from build123d import *

# Parameters (mm, degrees)
SKETCH1_R            = 10
BOSS_EXTRUDE1_DEPTH  = 340
SKETCH2_R            = 5
CUT_EXTRUDE1_DEPTH   = 330
BOSS_EXTRUDE2_START  = -10
SKETCH3_R            = 10
BOSS_EXTRUDE2_DEPTH  = 50
BOSS_EXTRUDE3_DEPTH  = 10
BOSS_EXTRUDE4_START  = -40
BOSS_EXTRUDE4_DEPTH  = 10
BOSS_EXTRUDE6_START  = 10
SKETCH5_W            = 35
SKETCH5_H            = 30
BOSS_EXTRUDE6_DEPTH  = 10
SKETCH6_W            = 35
SKETCH6_H            = 30
BOSS_EXTRUDE8_DEPTH  = 11
SKETCH7_R            = 6
CUT_EXTRUDE2_DEPTH   = 21
SKETCH8_R            = 2.5
BOSS_EXTRUDE9_DEPTH  = 4
SKETCH9_R            = 10
SKETCH9_R_2          = 7.5
SKETCH9_R_3          = 2.5
CUT_EXTRUDE3_DEPTH   = 3
SKETCH10_R           = 2
BOSS_EXTRUDE10_DEPTH = 5


with BuildPart() as part:
    # Sketch1 → Boss-Extrude1 (new body)
    with BuildSketch(Plane.XY):
        Circle(SKETCH1_R)
    extrude(amount=BOSS_EXTRUDE1_DEPTH)

    # Sketch2 → Cut-Extrude1 (cut)
    with BuildSketch(Plane.XY.offset(340)):
        Circle(SKETCH2_R)
    extrude(amount=-CUT_EXTRUDE1_DEPTH, mode=Mode.SUBTRACT)

    # Sketch3 → Boss-Extrude2 (add)
    with BuildSketch(Plane(origin=(0, 0, 0), x_dir=(-1, 0, 0), z_dir=(0, 0, -1)).offset(BOSS_EXTRUDE2_START)):
        Polygon((17.320508076, 0), (8.660254038, 15), (-8.660254038, 15), (-17.320508076, 0), (-8.660254038, -15), (8.660254038, -15), align=None)
        Circle(SKETCH3_R, mode=Mode.SUBTRACT)
    extrude(amount=-BOSS_EXTRUDE2_DEPTH)

    # Sketch4 → Boss-Extrude3 (add)
    with BuildSketch(Plane(origin=(0, 0, 10), x_dir=(-1, 0, 0), z_dir=(0, 0, -1))):
        Polygon((-9.526279442, -16.5), (9.526279442, -16.5), (19.052558883, 0), (9.526279442, 16.5), (-9.526279442, 16.5), (-19.052558883, 0), align=None)
        Polygon((8.660254038, 15), (-8.660254038, 15), (-17.320508076, 0), (-8.660254038, -15), (8.660254038, -15), (17.320508076, 0), align=None, mode=Mode.SUBTRACT)
    extrude(amount=-BOSS_EXTRUDE3_DEPTH)

    # Sketch4_2 → Boss-Extrude4 (add)
    with BuildSketch(Plane(origin=(0, 0, 10), x_dir=(-1, 0, 0), z_dir=(0, 0, -1)).offset(BOSS_EXTRUDE4_START)):
        Polygon((-9.526279442, -16.5), (9.526279442, -16.5), (19.052558883, 0), (9.526279442, 16.5), (-9.526279442, 16.5), (-19.052558883, 0), align=None)
        Polygon((8.660254038, 15), (-8.660254038, 15), (-17.320508076, 0), (-8.660254038, -15), (8.660254038, -15), (17.320508076, 0), align=None, mode=Mode.SUBTRACT)
    extrude(amount=-BOSS_EXTRUDE4_DEPTH)



with BuildPart() as body_2:
    # Sketch5 → Boss-Extrude6 (new body)
    with BuildSketch(Plane(origin=(10, 0, 0), x_dir=(0, 0, -1), z_dir=(1, 0, 0)).offset(BOSS_EXTRUDE6_START)):
        with Locations((-77.5, 1.5)):
            Rectangle(SKETCH5_W, SKETCH5_H)
    extrude(amount=BOSS_EXTRUDE6_DEPTH)


with BuildPart() as part_1:
    add(part.part)

    add(body_2.part)  # Boss-Extrude8 merges body 2
    # Sketch6 → Boss-Extrude8 (add)
    with BuildSketch(Plane.ZY.offset(-20)):
        with Locations((77.5, 1.5)):
            Rectangle(SKETCH6_W, SKETCH6_H)
    extrude(amount=BOSS_EXTRUDE8_DEPTH)

    # Sketch7 → Cut-Extrude2 (cut)
    with BuildSketch(Plane(origin=(0, 16.5, 0), x_dir=(1, 0, 0), z_dir=(0, 1, 0))):
        with Locations((19.5, -85)):
            Circle(SKETCH7_R)
    extrude(amount=-CUT_EXTRUDE2_DEPTH, mode=Mode.SUBTRACT)

    # Sketch8 → Boss-Extrude9 (add)
    with BuildSketch(Plane.ZY.offset(-9)):
        with Locations((90, 11.5)):
            Circle(SKETCH8_R)
    extrude(amount=BOSS_EXTRUDE9_DEPTH)

    # Sketch9 → Cut-Extrude3 (cut)
    with BuildSketch(Plane(origin=(30, 0, 0), x_dir=(0, 0, -1), z_dir=(1, 0, 0))):
        with Locations((-83, 4.5)):
            Circle(SKETCH9_R)
        with Locations((-83, 4.5)):
            Circle(SKETCH9_R_2, mode=Mode.SUBTRACT)
        with Locations((-83, 4.5)):
            Circle(SKETCH9_R_3)
    extrude(amount=-CUT_EXTRUDE3_DEPTH, mode=Mode.SUBTRACT)

    # Sketch10 → Boss-Extrude10 (add)
    with BuildSketch(Plane(origin=(30, 0, 0), x_dir=(0, 0, -1), z_dir=(1, 0, 0))):
        with Locations((-92, 13.5)):
            Circle(SKETCH10_R)
    extrude(amount=BOSS_EXTRUDE10_DEPTH)


solid = part_1.part
Read the model definition and answer for the solid it produces. Units are mm, in the model's axes. A direction names the side the tool comes from. Give positions to 0.01 mm unless a question says otherwise; leave off trailing zeros. Write each loop counter-clockwise with the first axis right and the second up, starting at its lowest first coordinate (ties: lowest second). Pieces come first, ordered by that corner, then holes. Notation, with made-up numbers: (-30.75, 84.5) -> (20.25, 84.5) arc R12 cw to (20.25, 94.5) -> close; hole circle Ø7 at (49, -22). An arc over 180 degrees is marked (long way). Answer as a JSON object with one key per item and string values. Group by question number.
1) Consider L1, parallel to Y at x = 28.3, z = 83; L2, parallel to X at y = 9, z = 85; L3, parallel to Z at x = -12.5, y = 10. Determine where each line is inside the solid, lowest interval first. Write a range as from..to.
2) A tool of negligible diameter and unlimited length cuts with its end or side. For faces 5 (the flat face through (14.36, -8.13, 14.93)), 6 (the flat face through (27, 11.2, 79.3)), 7 (the flat face through (0, 0, 10)), 8 (the flat face through (-14, 6.2, 50)), from which of +Z, -Z, +X, -X, +Y, -Y can it reach the whole face along a straight path? Write none if from no direction.
3) Find section A-A (z = 273). Write down the section's boundary in (x, y).
4) Each of these flat-tipped pins is pushed along its axis until it touches: P1, Ø3, axis at x = -6.5, z = 114, coming from the -Y side; P2, Ø12, axis at y = -5, z = 228, coming from the +X side; P3, Ø2.5, axis at y = 4.5, z = 83, coming from the +X side; P4, Ø4, axis at x = 13.5, z = 138, coming from the -Y side. Where does it stop, or does it pass through?
5) The mould has two halves that part along X. Classify faces 1 (the flat face through (13.05, -7.4, 34.79)), 2 (the flat face through (-14.36, 8.13, 14.93)), 3 (the flat face through (0, -16.5, 55)), 4 (the flat face through (9, 11, 77)): +X half, -X half, draft (parallel to the pull), parting line (faces both ways), or undercut.
Values follow:
{
 "1": {"L1": "y = -13.5..-5.5, -3..2, 7..12, 14.5..16.5", "L2": "x = -4.36..4.36, 9..13.5, 25.5..30", "L3": "z = 10..20, 50..60"},
 "2": {"face 5": "-Z, +X, -Y", "face 6": "+X", "face 7": "+Z", "face 8": "none"},
 "3": {"outline": "circle Ø20 at (0, 0); hole circle Ø10 at (0, 0)"},
 "4": {"P1": "stops at y = -8.66", "P2": "stops at x = 10", "P3": "stops at x = 27", "P4": "passes through"},
 "5": {"face 1": "+X half", "face 2": "-X half", "face 3": "draft", "face 4": "undercut"}
}
